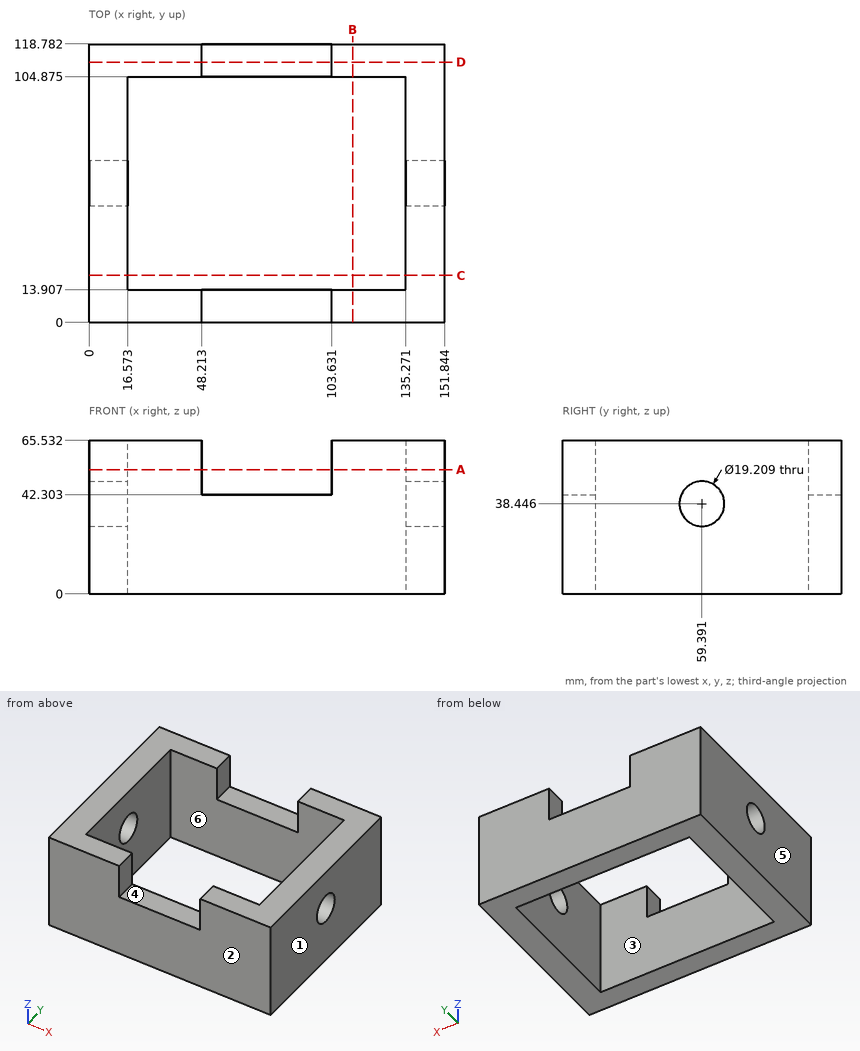
Check sheet for the drawn part. Datum: minimum x, y, z corner. Units: mm. A direction names the side the tool comes from. Round coordinates to 2 decimals unless told otherwise and drop trailing zeros. Loops run counter-clockwise (first coordinate to the right, second up) from the corner with the lowest first, then second, coordinate; pieces in that order, holes last. Notation, with made-up numbers: (-2.5, 8) - (11.5, 8) arc R30 ccw to (11.5, 31) - close; hole circle Ø8 at (13.5, 42.25). An arc over 180 degrees is marked (long way). Write item = value, one per line. Start each with the question number.
1. Thickness scan on line 1 (X direction, y = 102, z = 36.5); line 2 (Y direction, x = 23.5, z = 52) (1 decimal); line 3 (X direction, y = 10, z = 45). Record the ranges inside material, lowest first.
2. Section check B-B on x = 112.5. Enter the section's corners in (y, z) (1 decimal).
3. Section check C-C on y = 20. Enter the section's corners in (x, z).
4. Set-up check for the marked faces 4, 5 and 6: record each of +Z, -Z, +X, -X, +Y, -Y from which the full face is reachable in a straight line by a thin tool's end or side.
5. Section check D-D on y = 111. Enter the section's corners in (x, z), then the cut area to 3 significant figures.
6. Section check A-A on z = 53. Enter the section's corners in (x, y) (1 decimal).
7. Mould release check, pull along X, two halves, no side actions. Record for the marked faces 1, 2 and 3: released by +X, released by -X, zero draft, split by the parting line, or undercut.
8. Depth check by flat-ended pin: pin 1 (7 mm diameter, centred on x = 75, y = 108.5, fed in from +Z). Enter the tip coordinate at first touch or a pass-through.
Working result:
q1.line_1 = 0 to 16.57, 135.27 to 151.84
q1.line_2 = 0 to 13.9, 104.9 to 118.8
q1.line_3 = 0 to 48.21, 103.63 to 151.84
q2.outline = (0, 0) - (13.9, 0) - (13.9, 65.5) - (0, 65.5) - close; (104.9, 0) - (118.8, 0) - (118.8, 65.5) - (104.9, 65.5) - close
q3.outline = (0, 0) - (16.57, 0) - (16.57, 65.53) - (0, 65.53) - close; (135.27, 0) - (151.84, 0) - (151.84, 65.53) - (135.27, 65.53) - close
q4.face_4 = +Z, +Y, -Y
q4.face_5 = +Z, -Z, -X, +Y, -Y
q4.face_6 = +Z, -Z
q5.outline = (0, 0) - (151.84, 0) - (151.84, 65.53) - (103.63, 65.53) - (103.63, 42.3) - (48.21, 42.3) - (48.21, 65.53) - (0, 65.53) - close
q5.area = 8,660 mm^2
q6.outline = (0, 0) - (48.2, 0) - (48.2, 13.9) - (16.6, 13.9) - (16.6, 104.9) - (48.2, 104.9) - (48.2, 118.8) - (0, 118.8) - close; (103.6, 0) - (151.8, 0) - (151.8, 118.8) - (103.6, 118.8) - (103.6, 104.9) - (135.3, 104.9) - (135.3, 13.9) - (103.6, 13.9) - close
q7.face_1 = released by +X
q7.face_2 = zero draft
q7.face_3 = undercut
q8.pin_1 = 42.3
